from build123d import *

# Parameters (mm, degrees)
F0_W         = 402
F0_H         = 41
F0_W_2       = 17.5
F0_H_2       = 14
F0_R         = 1.6
F0_W_3       = 28
F0_H_3       = 20.8
F0_W_4       = 19.6
F0_H_4       = 10.9
F0_R_2       = 4.35
F1_DEPTH     = 1.1
F2_W         = 1.1
F2_H         = 25.2
F3_DEPTH     = 10.1
F4_W         = 402
F4_H         = 1.1
F5_DEPTH     = 255
F7_D         = 3.2
F9_D         = 3.2
F10_T1_DEPTH = 408.1720391711
F10_T3_DEPTH = 262.2720391711


# Not quite as in the source:
# - a fillet or chamfer that OpenCascade refuses, or shapes differently, is made with other operations: its cross-section is extruded or revolved along the edge and cut away or added


with BuildPart() as f1:
    # F0 (on Front) → F1 (new body)
    with BuildSketch(Plane.XZ):
        with Locations((201, -20.5)):
            Rectangle(F0_W, F0_H)
        with Locations((120, -26.8)):
            Rectangle(F0_W_2, F0_H_2, mode=Mode.SUBTRACT)
        with Locations((318.65, -26.25)):
            Circle(F0_R, mode=Mode.SUBTRACT)
        with Locations((331.35, -26.25)):
            Circle(F0_R, mode=Mode.SUBTRACT)
        with Locations((26, -19.9)):
            Circle(F0_R, mode=Mode.SUBTRACT)
        with Locations((46, -19.9)):
            Rectangle(F0_W_3, F0_H_3, mode=Mode.SUBTRACT)
        with Locations((66, -19.9)):
            Circle(F0_R, mode=Mode.SUBTRACT)
        with BuildLine():
            ThreePointArc((141.75, -9.65), (144, -7.4), (146.25, -9.65))
            Line((146.25, -9.65), (146.25, -30.15))
            ThreePointArc((146.25, -30.15), (144, -32.4), (141.75, -30.15))
            Line((141.75, -30.15), (141.75, -9.65))
        make_face(mode=Mode.SUBTRACT)
        with BuildLine():
            ThreePointArc((153.75, -9.65), (156, -7.4), (158.25, -9.65))
            Line((158.25, -9.65), (158.25, -30.15))
            ThreePointArc((158.25, -30.15), (156, -32.4), (153.75, -30.15))
            Line((153.75, -30.15), (153.75, -9.65))
        make_face(mode=Mode.SUBTRACT)
        with BuildLine():
            ThreePointArc((165.75, -9.65), (168, -7.4), (170.25, -9.65))
            Line((170.25, -9.65), (170.25, -30.15))
            ThreePointArc((170.25, -30.15), (168, -32.4), (165.75, -30.15))
            Line((165.75, -30.15), (165.75, -9.65))
        make_face(mode=Mode.SUBTRACT)
        with BuildLine():
            ThreePointArc((177.75, -9.65), (180, -7.4), (182.25, -9.65))
            Line((182.25, -9.65), (182.25, -30.15))
            ThreePointArc((182.25, -30.15), (180, -32.4), (177.75, -30.15))
            Line((177.75, -30.15), (177.75, -9.65))
        make_face(mode=Mode.SUBTRACT)
        with BuildLine():
            ThreePointArc((189.75, -9.65), (192, -7.4), (194.25, -9.65))
            Line((194.25, -9.65), (194.25, -30.15))
            ThreePointArc((194.25, -30.15), (192, -32.4), (189.75, -30.15))
            Line((189.75, -30.15), (189.75, -9.65))
        make_face(mode=Mode.SUBTRACT)
        with BuildLine():
            ThreePointArc((201.75, -9.65), (204, -7.4), (206.25, -9.65))
            Line((206.25, -9.65), (206.25, -30.15))
            ThreePointArc((206.25, -30.15), (204, -32.4), (201.75, -30.15))
            Line((201.75, -30.15), (201.75, -9.65))
        make_face(mode=Mode.SUBTRACT)
        with BuildLine():
            ThreePointArc((213.75, -9.65), (216, -7.4), (218.25, -9.65))
            Line((218.25, -9.65), (218.25, -30.15))
            ThreePointArc((218.25, -30.15), (216, -32.4), (213.75, -30.15))
            Line((213.75, -30.15), (213.75, -9.65))
        make_face(mode=Mode.SUBTRACT)
        with BuildLine():
            ThreePointArc((225.75, -9.65), (228, -7.4), (230.25, -9.65))
            Line((230.25, -9.65), (230.25, -30.15))
            ThreePointArc((230.25, -30.15), (228, -32.4), (225.75, -30.15))
            Line((225.75, -30.15), (225.75, -9.65))
        make_face(mode=Mode.SUBTRACT)
        with BuildLine():
            ThreePointArc((237.75, -9.65), (240, -7.4), (242.25, -9.65))
            Line((242.25, -9.65), (242.25, -30.15))
            ThreePointArc((242.25, -30.15), (240, -32.4), (237.75, -30.15))
            Line((237.75, -30.15), (237.75, -9.65))
        make_face(mode=Mode.SUBTRACT)
        with Locations((257.3, -19.9)):
            Circle(F0_R, mode=Mode.SUBTRACT)
        with Locations((269.8, -19.9)):
            Rectangle(F0_W_4, F0_H_4, mode=Mode.SUBTRACT)
        with Locations((282.3, -19.9)):
            Circle(F0_R, mode=Mode.SUBTRACT)
        with Locations((325, -19.9)):
            Circle(F0_R_2, mode=Mode.SUBTRACT)
        with Locations((318.65, -13.55)):
            Circle(F0_R, mode=Mode.SUBTRACT)
        with Locations((331.35, -13.55)):
            Circle(F0_R, mode=Mode.SUBTRACT)
    extrude(amount=F1_DEPTH)

    # F2 (on face) → F3 (join)
    with BuildSketch(Plane(origin=(0, 0, 0), x_dir=(-1, 0, 0), z_dir=(0, 1, 0))):
        with Locations((-401.45, -20.5)):
            Rectangle(F2_W, F2_H)
        with Locations((-0.55, -20.5)):
            Rectangle(F2_W, F2_H)
    extrude(amount=F3_DEPTH)

    # F4 (on face) → F5 (join)
    with BuildSketch(Plane(origin=(0, 0, 0), x_dir=(-1, 0, 0), z_dir=(0, 1, 0))):
        with Locations((-201, -40.45)):
            Rectangle(F4_W, F4_H)
    extrude(amount=F5_DEPTH)

    # F7 (through all)
    with Locations(Plane.XY.offset(-39.9)):
        with Locations((20.5, 90), (65.5, 90), (65.5, 176), (20.5, 176)):
            Hole(F7_D / 2)

    # F9 (through all)
    with Locations(Plane.XY.offset(-39.9)):
        with Locations((106.95, 6), (106.95, 78), (218.95, 6), (218.95, 78)):
            Hole(F9_D / 2)

    # F10: chamfer of 1.2 on 12 edges, made by hand

    # F10_s2 → F10_t1 (cut)
    with BuildSketch(Plane.YZ.offset(-3.0860195856)):
        Polygon((-1.1, -39.8), (0.1, -41), (-1.1, -41), align=None)
        Polygon((253.8, -41), (255, -39.8), (255, -41), align=None)
    extrude(amount=F10_T1_DEPTH, mode=Mode.SUBTRACT)

    # F10_s4 → F10_t3 (cut)
    with BuildSketch(Plane.XZ.offset(-258.0860195856)):
        Polygon((0, -39.8), (1.2, -41), (0, -41), align=None)
        Polygon((402, -39.8), (400.8, -41), (402, -41), align=None)
    extrude(amount=F10_T3_DEPTH, mode=Mode.SUBTRACT)

    # F10_s5 → F10_t6 (revolve, cut)
    with BuildSketch(Plane.XZ.offset(-6)):
        Polygon((109.75, -41), (108.55, -39.8), (108.55, -41), align=None)
    revolve(axis=Axis((106.95, 6, -41), (0, 0, 1)), mode=Mode.SUBTRACT)

    # F10_s7 → F10_t8 (revolve, cut)
    with BuildSketch(Plane.XZ.offset(-90)):
        Polygon((23.3, -41), (22.1, -39.8), (22.1, -41), align=None)
    revolve(axis=Axis((20.5, 90, -41), (0, 0, 1)), mode=Mode.SUBTRACT)

    # F10_s9 → F10_t10 (revolve, cut)
    with BuildSketch(Plane.XZ.offset(-90)):
        Polygon((68.3, -41), (67.1, -39.8), (67.1, -41), align=None)
    revolve(axis=Axis((65.5, 90, -41), (0, 0, 1)), mode=Mode.SUBTRACT)

    # F10_s11 → F10_t12 (revolve, cut)
    with BuildSketch(Plane.XZ.offset(-78)):
        Polygon((109.75, -41), (108.55, -39.8), (108.55, -41), align=None)
    revolve(axis=Axis((106.95, 78, -41), (0, 0, 1)), mode=Mode.SUBTRACT)

    # F10_s13 → F10_t14 (revolve, cut)
    with BuildSketch(Plane.XZ.offset(-6)):
        Polygon((221.75, -41), (220.55, -39.8), (220.55, -41), align=None)
    revolve(axis=Axis((218.95, 6, -41), (0, 0, 1)), mode=Mode.SUBTRACT)

    # F10_s15 → F10_t16 (revolve, cut)
    with BuildSketch(Plane.XZ.offset(-78)):
        Polygon((221.75, -41), (220.55, -39.8), (220.55, -41), align=None)
    revolve(axis=Axis((218.95, 78, -41), (0, 0, 1)), mode=Mode.SUBTRACT)

    # F10_s17 → F10_t18 (revolve, cut)
    with BuildSketch(Plane.XZ.offset(-176)):
        Polygon((23.3, -41), (22.1, -39.8), (22.1, -41), align=None)
    revolve(axis=Axis((20.5, 176, -41), (0, 0, 1)), mode=Mode.SUBTRACT)

    # F10_s19 → F10_t20 (revolve, cut)
    with BuildSketch(Plane.XZ.offset(-176)):
        Polygon((68.3, -41), (67.1, -39.8), (67.1, -41), align=None)
    revolve(axis=Axis((65.5, 176, -41), (0, 0, 1)), mode=Mode.SUBTRACT)


solid = f1.part
Check sheet for the modelled part. Datum: model origin and axes. Units: mm. A direction names the side the tool comes from. Coordinates: 2 decimals unless noted, no trailing zeros. Loops run counter-clockwise (first coordinate to the right, second up) from the corner with the lowest first, then second, coordinate; pieces in that order, holes last. Notation, with made-up numbers: (36, -13) -> (77, -13) arc R4 ccw to (77, -6) -> close; hole circle Ø3 at (61.5, 33). An arc over 180 degrees is marked (long way). Write item = value, one per line. Start each with the question number.
1. Section check A-A on x = 292. Record the cut outline in (y, z).
2. Section check B-B on y = 103. Record the cut outline in (x, z).
3. Depth check by flat-ended pin: P1, Ø2, axis at x = 160.5, y = 59, coming from the +Z side; P2, Ø2.5, axis at x = 318.65, z = -26.25, coming from the -Y side (1 decimal); P3, Ø3.5, axis at x = 282.3, z = -19.9, coming from the +Y side; P4, Ø0.9, axis at x = 117.5, y = -0.5, coming from the -Z side. Enter the tip coordinate at first touch or a pass-through.
4. Tool access check on faces 1 (the flat face through (400.9, 5, -21)), 2 (the flat face through (402, 4, -20)). Record the directions out of +Z, -Z, +X, -X, +Y, -Y that give a thin tool (end or side, any length) a straight path to the whole face; none if there is none.
5. Material ranges on line 1 (Y direction, x = 75.5, z = -3); line 2 (Z direction, x = 263, y = 231.5); line 3 (Z direction, x = 331.35, y = -0.45), recorded low to high.
6. Draft check along X on faces 3 (the flat face through (198, -1.1, -20)), 4 (the cylindrical face through (329.15, -0.54, -18.59)), 5 (the flat face through (0, 4, -20)). Enter one of: released by +X, released by -X, zero draft, split by the parting line, or undercut.
Responses:
q1.outline = (-1.1, -39.8) -> (0.1, -41) -> (253.8, -41) -> (254.9, -39.9) -> (0, -39.9) -> (0, 0) -> (-1.1, 0) -> close
q2.outline = (0.1, -39.9) -> (1.2, -41) -> (400.8, -41) -> (401.9, -39.9) -> close
q3.P1 = -39.9
q3.P2 = through
q3.P3 = 0
q3.P4 = -40.85
q4.face_1 = +Z, +Y
q4.face_2 = +Z, -Z, +X, +Y, -Y
q5.line_1 = -1.1 to 0
q5.line_2 = -41 to -39.9
q5.line_3 = -40.45 to -27.85, -24.65 to -15.15, -11.95 to 0
q6.face_3 = zero draft
q6.face_4 = undercut
q6.face_5 = released by -X
